Geometry: final body of the model. Coordinates: model frame, mm. Give positions to 0.01 mm unless a question says otherwise; leave off trailing zeros.
```python
from build123d import *

# Parameters (mm, degrees)
F0_W     = 130
F0_H     = 180
F1_DEPTH = 4
F2_R     = 3
F3_W     = 124
F3_H     = 174
F4_DEPTH = 1
F5_R     = 2


with BuildPart() as f1:
    # F0 (on Front) → F1 (new body)
    with BuildSketch(Plane.XZ):
        with Locations((-17.656866, 35.967222)):
            Rectangle(F0_W, F0_H)
    extrude(amount=F1_DEPTH)

    # F2
    f2_edges = [f1.edges().sort_by_distance(p)[0] for p in [
        (-82.656866, -2, 125.967222),
        (-82.656866, -2, -54.032778),
        (47.343134, -2, -54.032778),
        (47.343134, -2, 125.967222),
    ]]
    fillet(f2_edges, radius=F2_R)

    # F3 (on face) → F4 (join)
    with BuildSketch(Plane.XZ.offset(4)):
        with Locations((-17.656866, 35.967222)):
            Rectangle(F3_W, F3_H)
    extrude(amount=F4_DEPTH)

    # F5
    f5_edges = [f1.edges().sort_by_distance(p)[0] for p in [
        (-79.656866, -4.5, 122.967222),
        (44.343134, -4.5, 122.967222),
        (-79.656866, -4.5, -51.032778),
        (44.343134, -4.5, -51.032778),
    ]]
    fillet(f5_edges, radius=F5_R)


solid = f1.part
```
Item 1: Pin query (flat end, axial travel): pin 1 Ø0.5 at (y, z) = (-4.5, 48.5) entering from -X. Return the tip coordinate at first contact, or that it passes through.
Found:
pin 1: stops at x = -79.66
Item 2: Line query: L1, parallel to X at y = -4.2, z = 8. Output: solid intervals per line, ascending.
Found:
L1: x = -79.66 to 44.34
Item 3: Pull-direction query (Z, two-part tool) for faces 1 (the face through (-19, -2, -54.033)), 2 (the face through (-19, 0, 37)), 3 (the face through (-19, -2, 125.967)); classes: +Z half, -Z half, draft (parallel to the pull), parting line (faces both ways), or undercut.
Found:
face 1: -Z half
face 2: draft
face 3: +Z half
